from build123d import *

# Parameters (mm, degrees)
CROQUIS1_R              = 1.5
SALIENTE_EXTRUIR1_DEPTH = 3


with BuildPart() as part:
    # Croquis1 → Saliente-Extruir1 (new body)
    with BuildSketch(Plane(origin=(0, 0, 0), x_dir=(1, 0, 0), z_dir=(0, 1, 0))):
        with BuildLine():
            Line((-35.322649353, -4.523785763), (-29.713798408, 25.866039525))
            Line((-29.713798408, 25.866039525), (-35.221795469, 52.273603799))
            Line((-35.221795469, 52.273603799), (-36.45117663, 78.681168073))
            ThreePointArc((-36.45117663, 78.681168073), (-34.470773885, 85.134483293), (-28.840989272, 88.859103754))
            Line((-28.840989272, 88.859103754), (0, 95.923167849))
            Line((0, 95.923167849), (28.745582144, 88.873347738))
            ThreePointArc((28.745582144, 88.873347738), (34.369430491, 85.153487685), (36.353462125, 78.709215227))
            Line((36.353462125, 78.709215227), (35.159044734, 52.307970662))
            Line((35.159044734, 52.307970662), (29.69822954, 25.906726097))
            Line((29.69822954, 25.906726097), (35.352965357, -4.492390106))
            Line((35.352965357, -4.492390106), (36.368027066, -26.718230301))
            ThreePointArc((36.368027066, -26.718230301), (34.398862632, -33.147130574), (28.803795931, -36.875883169))
            Line((28.803795931, -36.875883169), (2.42535625, -43.470493089))
            ThreePointArc((2.42535625, -43.470493089), (0, -43.769068087), (-2.42535625, -43.470493089))
            Line((-2.42535625, -43.470493089), (-28.730703822, -36.894156196))
            ThreePointArc((-28.730703822, -36.894156196), (-34.320110297, -33.172996946), (-36.295781209, -26.755426116))
            Line((-36.295781209, -26.755426116), (-35.322649353, -4.523785763))
        make_face()
        with Locations(Location((-20.692659667, 67.660143415, 0), (0, 0, 270))):
            Circle(CROQUIS1_R, mode=Mode.SUBTRACT)
        with Locations(Location((20.730030015, 67.612237294, 0), (0, 0, 270))):
            Circle(CROQUIS1_R, mode=Mode.SUBTRACT)
        with Locations(Location((-20.750709845, -15.848615277, 0), (0, 0, 270))):
            Circle(CROQUIS1_R, mode=Mode.SUBTRACT)
        with Locations(Location((20.809934934, -15.806357426, 0), (0, 0, 270))):
            Circle(CROQUIS1_R, mode=Mode.SUBTRACT)
    extrude(amount=SALIENTE_EXTRUIR1_DEPTH)


solid = part.part
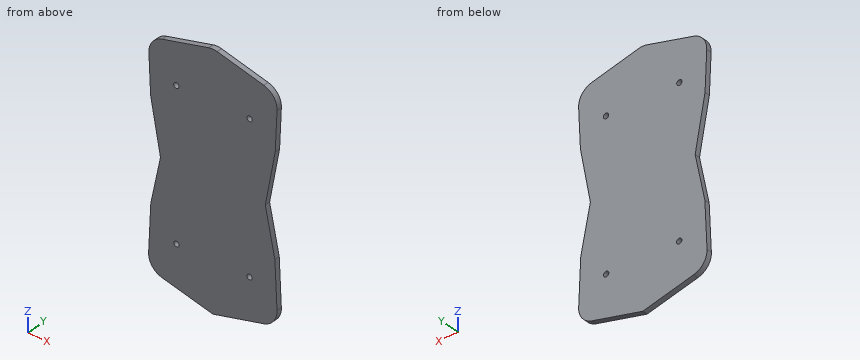
The model under review builds one solid part; all positions refer to its coordinate system, in mm. Coordinates: 2 decimals unless noted, no trailing zeros. Loops run counter-clockwise (first coordinate to the right, second up) from the corner with the lowest first, then second, coordinate; pieces in that order, holes last. Notation, with made-up numbers: (57.25, 72) -> (83.25, 72) arc R19 cw to (83.25, 98) -> close; hole circle Ø2 at (73.25, 70.5). An arc over 180 degrees is marked (long way). Use a Markdown table: item, result. Add a question column.
1. To check wall thickness, follow line 1 (X direction, y = 0.25, z = 5); line 2 (X direction, y = 1.25, z = -31); line 3 (Z direction, x = 6.5, y = 2.8). State the ranges of each line that lie inside material, in increasing order.
2. Add section B-B on z = -7.5. Write out the cut boundary in (x, y), plus the area to 3 significant figures.
3. Add section C-C on x = -14.5. Write out the cut boundary in (y, z).
4. Clearance check with flat-ended pins moving along their axes: pin 1 Ø1.5 at (y, z) = (1, -74.5) entering from +X; pin 2 Ø2.5 at (x, z) = (20.81, 15.81) entering from -Y; pin 3 Ø1.5 at (x, y) = (23, 1.5) entering from +Z. State where each tip first meets the part, or that it passes through.
5. Add section A-A on y = 0.7. Write out the cut boundary in (x, z).
Returned:
| question | item | result |
|---|---|---|
| 1 | line 1 | x = -35.34 to 35.38 |
| 1 | line 2 | x = -30.78 to 30.75 |
| 1 | line 3 | z = -94.33 to 42.45 |
| 2 | outline | (-33.1, 0) -> (33.12, 0) -> (33.12, 3) -> (-33.1, 3) -> close |
| 2 | area | 199 mm² |
| 3 | outline | (0, -92.37) -> (3, -92.37) -> (3, 40.45) -> (0, 40.45) -> close |
| 4 | pin 1 | stops at x = 36.2 |
| 4 | pin 2 | passes through |
| 4 | pin 3 | stops at z = 38.51 |
| 5 | outline | (-36.45, -78.68) arc R10 ccw to (-28.84, -88.86) -> (0, -95.92) -> (28.75, -88.87) arc R10 ccw to (36.35, -78.71) -> (35.16, -52.31) -> (29.7, -25.91) -> (35.35, 4.49) -> (36.37, 26.72) arc R10 ccw to (28.8, 36.88) -> (2.43, 43.47) arc R10 ccw to (-2.43, 43.47) -> (-28.73, 36.89) arc R10 ccw to (-36.3, 26.76) -> (-35.32, 4.52) -> (-29.71, -25.87) -> (-35.22, -52.27) -> close; hole circle Ø3 at (-20.75, 15.85); hole circle Ø3 at (-20.69, -67.66); hole circle Ø3 at (20.73, -67.61); hole circle Ø3 at (20.81, 15.81) |
